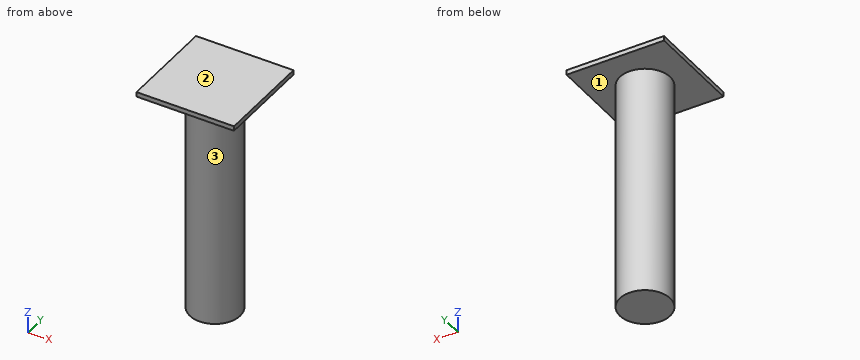
```python
from build123d import *

# Parameters (mm, degrees)
F0_R     = 16
F1_DEPTH = 150
F2_W     = 62
F2_H     = 62
F3_DEPTH = 3


with BuildPart() as f1:
    # F0 (on Top) → F1 (new body)
    with BuildSketch(Plane.XY):
        Circle(F0_R)
    extrude(amount=-F1_DEPTH)

    # F2 (on Top) → F3 (join)
    with BuildSketch(Plane.XY):
        Rectangle(F2_W, F2_H)
    extrude(amount=-F3_DEPTH)


solid = f1.part
```
CAD build for the part. Positions are in the model's coordinates, mm. Face numbers are marked on the shaded views. Coordinates: 2 decimals unless noted, no trailing zeros. Order: outer loops, then holes, each group sorted by start corner. A loop starts at its lowest first (then second) coordinate and runs counter-clockwise, first axis right, second up. Notation, with made-up numbers: (-3, -1.75) -> (45, -1.75) arc R20 cw to (45, 3.25) -> close; hole circle Ø7 at (58, 37.5). An arc over 180 degrees is marked (long way). Use one line per item in the form item = value. Start each with the question number.
1) Band-saw the part on C-C on z = -81. Give the cut face in (x, y), then the cut area to 3 significant figures.
2) Band-saw the part on A-A on y = 0. Give the cut face in (x, z).
3) Pull direction Z, two halves, no side cores. Call the marked faces 1, 2 and 3: +Z half, -Z half, draft (parallel to the pull), parting line (faces both ways), or undercut.
4) Drill centre lines: L1, parallel to Y at x = 0.5, z = -118.5; L2, parallel to Z at x = -15, y = -25.5; L3, parallel to X at y = -11.5, z = -53. Where is each one in solid material? Low to high. Write a range as [from, to].
5) Band-saw the part on D-D on x = 23. Give the cut face in (y, z).
6) Drop flat-ended pins along their axis: pin 1 (1.5 mm diameter, centred on y = 6, z = -42, fed in from -X); pin 2 (5 mm diameter, centred on x = 4.5, z = -89.5, fed in from +Y); pin 3 (6 mm diameter, centred on y = -4, z = -117, fed in from +X). Give the stop position or say it passes through.
Entries:
q1.outline = circle Ø32 at (0, 0)
q1.area = 804 mm2
q2.outline = (-31, -3) -> (-16, -3) -> (-16, -150) -> (16, -150) -> (16, -3) -> (31, -3) -> (31, 0) -> (-31, 0) -> close
q3.face_1 = -Z half
q3.face_2 = +Z half
q3.face_3 = draft
q4.L1 = [-15.99, 15.99]
q4.L2 = [-3, 0]
q4.L3 = [-11.12, 11.12]
q5.outline = (-31, -3) -> (31, -3) -> (31, 0) -> (-31, 0) -> close
q6.pin_1 = -15.11
q6.pin_2 = 15.87
q6.pin_3 = 15.97
